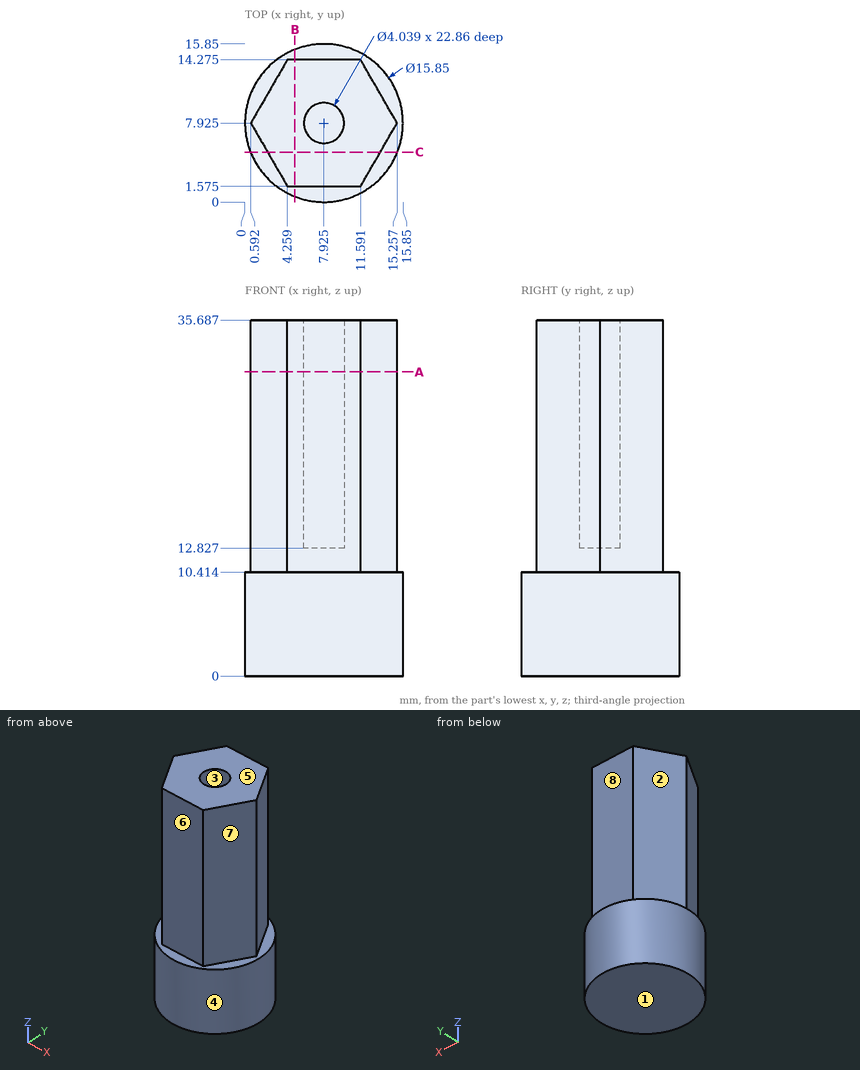
Study the drawing (mm; zero at the part's minimum x, y, z) and answer. A direction names the side the tool comes from. Give positions to 0.01 mm unless a question says otherwise; leave off trailing zeros. Order: outer loops, then holes, each group sorted by start corner. A loop starts at its lowest first (then second) coordinate and runs counter-clockwise, first axis right, second up. Notation, with made-up numbers: (75.25, -8) -> (114.25, -8) arc R16 ccw to (114.25, 3) -> close; hole circle Ø1 at (60, 72). An arc over 180 degrees is marked (long way). Write item = value, one per line.
1. Straight lines are drawn through the part: line 1 along X through (y, z) = (6.75, 25) (1 decimal); line 2 along Y through (x, z) = (10.5, 17) (1 decimal); line 3 along X through (y, z) = (8, 4). For each, find the intervals that lie inside material, in ascending order.
Numbers:
line_1 = 1.3 to 6.3, 9.6 to 14.6
line_2 = 1.6 to 14.3
line_3 = 0 to 15.85
2. The mould has two halves that part along Y. Classify the marked faces 1, 2 and 3: +Y half, -Y half, draft (parallel to the pull), parting line (faces both ways), or undercut.
Numbers:
face_1 = draft
face_2 = +Y half
face_3 = undercut
3. Given pin 1 (5 mm diameter, centred on y = 12.5, z = 25, fed in from -X); pin 2 (2 mm diameter, centred on x = 2, z = 17, fed in from +Y) (1 decimal); pin 3 (2 mm diameter, centred on x = 9.5, z = 23, fed in from -Y) (1 decimal), each flat-ended and moving along its own axis, determine where each tip first touches the part or whether it passes through.
Numbers:
pin_1 = 1.79
pin_2 = 12.1
pin_3 = 1.6
4. A cutting plane is placed at B-B, the plane x = 5. Write down the section's boundary in (y, z) (1 decimal).
Numbers:
outline = (0.6, 0) -> (15.3, 0) -> (15.3, 10.4) -> (14.3, 10.4) -> (14.3, 35.7) -> (1.6, 35.7) -> (1.6, 10.4) -> (0.6, 10.4) -> close
5. A cutting plane is placed at C-C, the plane y = 5. Write down the section's boundary in (x, z), and give its area (3 significant figures).
Numbers:
outline = (0.56, 0) -> (15.29, 0) -> (15.29, 10.41) -> (13.57, 10.41) -> (13.57, 35.69) -> (2.28, 35.69) -> (2.28, 10.41) -> (0.56, 10.41) -> close
area = 439 mm²
6. For the marked faces 4, 5, 6, 7 and 8, determine the directions among +Z, -Z, +X, -X, +Y, -Y from which every point of the face is accessible in a straight line to the end or side of a thin tool.
Numbers:
face_4 = +Z, -Z
face_5 = +Z, +X, -X, +Y, -Y
face_6 = +Z, +X, -X, -Y
face_7 = +Z, +X, -Y
face_8 = +Z, +X, -X, +Y
7. A cutting plane is placed at A-A, the plane z = 30.5. Write down the section's boundary in (x, y) (1 decimal), and give its area (3 significant figures).
Numbers:
outline = (0.6, 7.9) -> (4.3, 1.6) -> (11.6, 1.6) -> (15.3, 7.9) -> (11.6, 14.3) -> (4.3, 14.3) -> close; hole circle Ø4 at (7.9, 7.9)
area = 127 mm²
